The listing builds one solid part. Answer for the finished solid, in the listing's coordinates (mm). A direction names the side the tool comes from. Give positions to 0.01 mm unless a question says otherwise; leave off trailing zeros. Loops run counter-clockwise (first coordinate to the right, second up) from the corner with the lowest first, then second, coordinate; pieces in that order, holes last. Notation, with made-up numbers: (-25, 79.25) - (10, 79.25) arc R19 ccw to (10, 95.25) - close; hole circle Ø8 at (8, 28.25). An arc over 180 degrees is marked (long way). Write item = value, one per line. Start each with the question number.
1) Which of the six approach directions +Z, -Z, +X, -X, +Y, -Y give full straight-line access (tool end or side, diameter ignored) to faces 1 (the flat face through (-4, 0, -8)), 2 (the flat face through (0, -4, -4)), 3 (the flat face through (0, -4, 68))?
2) The part is cut by section B-B on x = 1. Write down the section's boundary in (y, z).
3) Consider probe 1 along Z at (x, y) = (4, -1.5); probe 2 along X at (y, z) = (0.25, 35.5); probe 3 along Y at (x, z) = (-4.25, 42.5). Determine where each line is inside the solid, lowest interval first.
4) The part is cut by section D-D on y = 4.5. Write down the section's boundary in (x, z).
5) Flat-ended cylindrical pins translate along their axes: P1, Ø1.6, axis at y = -4.5, z = -5, coming from the +X side; P2, Ø3, axis at y = -2.5, z = 0, coming from the +X side; P3, Ø1.5, axis at x = 4.5, z = 20, coming from the +Y side. Find the tip coordinate at first contact, or state that the pin passes through.
6) The part is cut by section A-A on y = 1.25. Write down the section's boundary in (x, z).
7) The part is cut by section C-C on z = 5. Write down the section's boundary in (x, y), plus the area to 3 significant figures.
from build123d import *
from build123d.topology import SkipClean

# Parameters (mm, degrees)
SKETCH1_R                                        = 5.5
SKETCH1_R_2                                      = 3.5
BOSS_EXTRUDE1_DLUGOSC_CALKOWITA_DEPTH            = 64.16
BOSS_EXTRUDE2_PRZEDLUZENIE_DO_MONTAZU_DEPTH      = 8
BOSS_EXTRUDE2_PRZEDLUZENIE_DO_MONTAZU_DEPTH_BACK = 72.16


with BuildPart() as part:
    # Sketch1 → Boss-Extrude1 dlugosc calkowita (new body)
    with BuildSketch(Plane.XY):
        Circle(SKETCH1_R)
        Circle(SKETCH1_R_2, mode=Mode.SUBTRACT)
    extrude(amount=BOSS_EXTRUDE1_DLUGOSC_CALKOWITA_DEPTH)

    # Sketch2 → Boss-Extrude2 przedluzenie do montazu (add, two sides: drawn at the far end of the back side and taken through both)
    with SkipClean():  # the faces are left unmerged after this step: merging them gives an invalid solid
        with BuildSketch(Plane(origin=(0, 0, 0), x_dir=(-1, 0, 0), z_dir=(0, 0, -1)).offset(-BOSS_EXTRUDE2_PRZEDLUZENIE_DO_MONTAZU_DEPTH_BACK)):
            with BuildLine():
                Line((0, 5.5), (0, 3.5))
                ThreePointArc((0, 3.5), (3.5, 0), (0, -3.5))
                Line((0, -3.5), (0, -5.5))
                ThreePointArc((0, -5.5), (5.5, 0), (0, 5.5))
            make_face()
        extrude(amount=BOSS_EXTRUDE2_PRZEDLUZENIE_DO_MONTAZU_DEPTH + BOSS_EXTRUDE2_PRZEDLUZENIE_DO_MONTAZU_DEPTH_BACK)
    add(part.part.scale(1), mode=Mode.REPLACE)  # the faces are merged on a copy


solid = part.part
Answer below:
q1.face_1 = -Z, +X, -X, +Y, -Y
q1.face_2 = -Z, +X, +Y, -Y
q1.face_3 = +Z, +X, +Y, -Y
q2.outline = (-5.41, 0) - (-3.35, 0) - (-3.35, 64.16) - (-5.41, 64.16) - close; (3.35, 0) - (5.41, 0) - (5.41, 64.16) - (3.35, 64.16) - close
q3.probe_1 = 0 to 64.16
q3.probe_2 = -5.49 to -3.49, 3.49 to 5.49
q3.probe_3 = -3.49 to 3.49
q4.outline = (-3.16, -8) - (0, -8) - (0, 0) - (3.16, 0) - (3.16, 64.16) - (0, 64.16) - (0, 72.16) - (-3.16, 72.16) - close
q5.P1 = 0
q5.P2 = 5.41
q5.P3 = 4.02
q6.outline = (-5.36, -8) - (-3.27, -8) - (-3.27, 72.16) - (-5.36, 72.16) - close; (3.27, 0) - (5.36, 0) - (5.36, 64.16) - (3.27, 64.16) - close
q7.outline = circle Ø11 at (0, 0); hole circle Ø7 at (0, 0)
q7.area = 56.5 mm2
